Source: CAD feature listing. Evaluate the final solid. Frame: model axes, mm. Face numbers are marked on the shaded views. A direction names the side the tool comes from. Give positions to 0.01 mm unless a question says otherwise; leave off trailing zeros. Write each loop counter-clockwise with the first axis right and the second up, starting at its lowest first coordinate (ties: lowest second). Pieces come first, ordered by that corner, then holes. Notation, with made-up numbers: (58, 63) -> (116, 63) arc R20 cw to (116, 72) -> close; hole circle Ø8 at (-4, 68). An arc over 180 degrees is marked (long way). Write item = value, one per line.
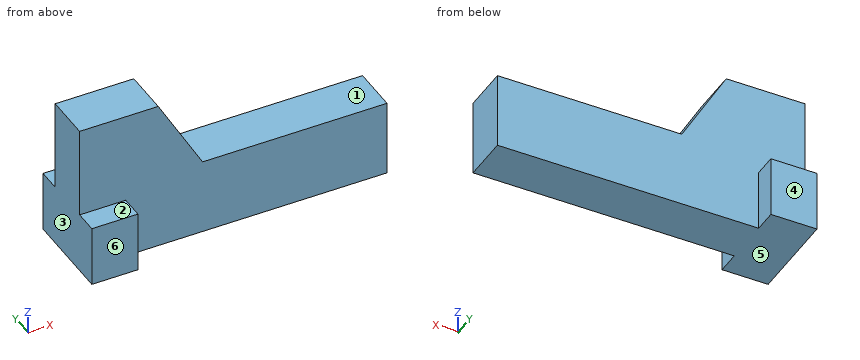
from build123d import *

# Parameters (mm, degrees)
F1_DEPTH = 19.05
F2_W     = 19.05
F2_H     = 25.4
F3_DEPTH = 9.525
F4_W     = 19.05
F4_H     = 25.4
F5_DEPTH = 9.525


with BuildPart() as f1:
    # F0 (on Front) → F1 (new body)
    with BuildSketch(Plane.XZ):
        Polygon((-49.55082, 26.919836), (-49.55082, -36.580164), (77.44918, -36.580164), (77.44918, -4.830164), (1.24918, -4.830164), (-17.081691, 26.919836), align=None)
    extrude(amount=F1_DEPTH)

    # F2 (on face) → F3 (join)
    with BuildSketch(Plane.XZ.offset(19.05)):
        with Locations((-40.02582, -23.880164)):
            Rectangle(F2_W, F2_H)
    extrude(amount=F3_DEPTH)

    # F4 (on face) → F5 (join)
    with BuildSketch(Plane(origin=(0, 0, 0), x_dir=(-1, 0, 0), z_dir=(0, 1, 0))):
        with Locations((40.02582, -23.880164)):
            Rectangle(F4_W, F4_H)
    extrude(amount=F5_DEPTH)


solid = f1.part
(1) Pull-direction query (Y, two-part tool) for the marked faces 4, 5 and 6; classes: pulls with the +Y half, pulls with the -Y half, needs draft (parallel to the pull), parting line crosses it, or undercut.
Values follow:
face_4 = pulls with the +Y half
face_5 = needs draft
face_6 = pulls with the -Y half
(2) Section query B-B (x = -27). Return loops of the section in (y, z).
Values follow:
outline = (-19.05, -36.58) -> (0, -36.58) -> (0, 26.92) -> (-19.05, 26.92) -> close
(3) First-contact query: pin 1 (10.5 mm diameter, centred on y = -25, z = -23, fed in from +X); pin 2 (5.5 mm diameter, centred on x = 31.5, y = -8, fed in from +Z); pin 3 (3 mm diameter, centred on x = -1.5, z = -8, fed in from -Y). Flat tips, straight axial feed; report the tip coordinate or a pass-through.
Values follow:
pin_1 = -30.5
pin_2 = -4.83
pin_3 = -19.05
(4) Section query A-A (z = -29.5). Return loops of the section in (x, y) (3 decimals).
Values follow:
outline = (-49.551, -28.575) -> (-30.501, -28.575) -> (-30.501, -19.05) -> (77.449, -19.05) -> (77.449, 0) -> (-30.501, 0) -> (-30.501, 9.525) -> (-49.551, 9.525) -> close
(5) Section query C-C (y = -26). Return loops of the section in (x, z), plus the area to 3 significant figures.
Values follow:
outline = (-49.55, -36.58) -> (-30.5, -36.58) -> (-30.5, -11.18) -> (-49.55, -11.18) -> close
area = 484 mm2
(6) Material intervals for line 1 (Y direction, x = -31.5, z = 7.5); line 2 (X direction, y = 7, z = -31); line 3 (Z direction, x = 69, y = -8.5), sorted ascending.
Values follow:
line_1 = -19.05 to 0
line_2 = -49.55 to -30.5
line_3 = -36.58 to -4.83
(7) Access query for the marked faces 1, 2 and 3. Directions: +Z, -Z, +X, -X, +Y, -Y. A direction counts if a zero-diameter tool reaches every point of the face in a straight line with its end or side. Return the directions, or none.
Values follow:
face_1 = +Z, +X, +Y, -Y
face_2 = +Z, +X, -X, -Y
face_3 = +Z, -Z, -X, +Y, -Y
(8) Section query D-D (y = -14). Return loops of the section in (x, z), plus the area to 3 significant figures.
Values follow:
outline = (-49.55, -36.58) -> (77.45, -36.58) -> (77.45, -4.83) -> (1.25, -4.83) -> (-17.08, 26.92) -> (-49.55, 26.92) -> close
area = 5,350 mm2
